from build123d import *

# Parameters (mm, degrees)
BOSS_EXTRUDE1_DEPTH = 50
SKETCH3_R           = 4.7625
CUT_EXTRUDE1_DEPTH  = 6.35


with BuildPart() as part:
    # Sketch1 → Boss-Extrude1 (new body)
    with BuildSketch(Plane.XY):
        Polygon((0, 0), (0, 15), (8, 15), (4, 11), (46, 11), (42, 15), (50, 15), (50, 0), align=None)
    extrude(amount=BOSS_EXTRUDE1_DEPTH)

    # Sketch2 → Revolve2 (revolve)
    with BuildSketch(Plane.XY.offset(25)):
        Polygon((50, 6), (50, 1), (62.5, 1), (62.5, -3), (79, -3), (79, 6), align=None)
    revolve(axis=Axis((50, 6, 25), (1, 0, 0)))

    # Sketch3 → Cut-Extrude1 (cut)
    with BuildSketch(Plane.XZ):
        with Locations((25, 25)):
            Circle(SKETCH3_R)
    extrude(amount=-CUT_EXTRUDE1_DEPTH, mode=Mode.SUBTRACT)


solid = part.part
Verification items for the finished model (mm, model axes). A direction names the side the tool comes from. Round coordinates to 2 decimals unless told otherwise and drop trailing zeros. Loops run counter-clockwise (first coordinate to the right, second up) from the corner with the lowest first, then second, coordinate; pieces in that order, holes last. Notation, with made-up numbers: (-32.75, 81) - (13.25, 81) arc R15 ccw to (13.25, 85) - close; hole circle Ø1 at (49.25, 40). An arc over 180 degrees is marked (long way). Use one line per item in the form item = value.
1. Section check A-A on x = 44. Record the cut outline in (y, z), and give its area (3 significant figures).
A:
outline = (0, 0) - (11, 0) - (11, 50) - (0, 50) - close; (13, 0) - (15, 0) - (15, 50) - (13, 50) - close
area = 650 mm²
2. Draft check along X on faces 1 (the flat face through (50, 13, 25)), 2 (the flat face through (79, 6, 25)), 3 (the flat face through (25, 11, 25)), 4 (the flat face through (25, 0, 19)). Enter one of: pulls with the +X half, pulls with the -X half, needs draft (parallel to the pull), parting line crosses it, or undercut.
A:
face_1 = undercut
face_2 = pulls with the +X half
face_3 = undercut
face_4 = needs draft
3. Gauge pin test, flat ends, axial feed: pin 1 Ø10 at (x, z) = (30, 43.5) entering from +Y; pin 2 Ø4 at (x, y) = (63, 2.5) entering from +Z; pin 3 Ø3 at (x, z) = (23, 27) entering from -Y. Record the tip position at first contact, or that the pin passes through.
A:
pin_1 = 11
pin_2 = 33.87
pin_3 = 6.35
4. Section check D-D on z = 4.5. Record the cut outline in (x, y), and give its area (3 significant figures).
A:
outline = (0, 0) - (50, 0) - (50, 15) - (42, 15) - (46, 11) - (4, 11) - (8, 15) - (0, 15) - close
area = 598 mm²
5. Section check C-C on x = 25. Record the cut outline in (y, z).
A:
outline = (0, 0) - (11, 0) - (11, 50) - (0, 50) - (0, 29.76) - (6.35, 29.76) - (6.35, 20.24) - (0, 20.24) - close
6. Scan lines: probe 1 along Z at (x, y) = (25, 3.5); probe 2 along X at (y, z) = (10, 32); probe 3 along X at (y, z) = (12.5, 19.5). Record each from-to range of solid material in increasing order.
A:
probe_1 = 0 to 20.24, 29.76 to 50
probe_2 = 0 to 50, 62.5 to 79
probe_3 = 0 to 5.5, 44.5 to 50, 62.5 to 79
7. Section check B-B on y = 3.5. Record the cut outline in (x, z) (1 decimal).
A:
outline = (0, 0) - (50, 0) - (50, 20.7) - (62.5, 20.7) - (62.5, 16.4) - (79, 16.4) - (79, 33.6) - (62.5, 33.6) - (62.5, 29.3) - (50, 29.3) - (50, 50) - (0, 50) - close; hole circle Ø9.5 at (25, 25)
8. Access from +Z, -Z, +X, -X, +Y, -Y to the whole of each face (thin tool, end or side, straight path). Record for faces 5 (the cylindrical face through (70.866, -2.584, 22.297)), 6 (the cylindrical face through (56.34, 7.08, 29.88)), 7 (the flat face through (25, 6.35, 25)).
A:
face_5 = +X
face_6 = none
face_7 = -Y
